Autodesk Inventor part; units mm, degrees
ref_plane "YZ Plane" through (0, 0, 0) normal (1, 0, 0) x (0, 1, 0)
ref_plane "XZ Plane" through (0, 0, 0) normal (0, 1, 0) x (-1, 0, 0)
ref_plane "XY Plane" through (0, 0, 0) normal (0, 0, 1) x (1, 0, 0)
sketch "Sketch1" plane through (0, 0, 0) normal (0, 0, 1) x (1, 0, 0)
  line L0 (0, 0) -> (7.0104, 0)
  line L1 (7.0104, 0) -> (7.0104, 3.9878)
  line L2 (7.0104, 3.9878) -> (0, 3.9878)
  line L3 (0, 3.9878) -> (0, 0)
  dimension "d0" = 7.0104
  dimension "d1" = 3.9878
extrude "Extrusion1" add sketch "Sketch1" against normal blind 1.0922
sketch "Sketch2" plane through (0, 0, -1.0922) normal (0, 0, -1) x (-1, 0, 0)
  line L0 (-7.0104, 0) -> (-7.0104, 3.9878)
  line L1 (-7.0104, 3.9878) -> (0, 3.9878)
  line L2 (-6.0071, 0.8001) -> (-1.0033, 0.8001)
  line L3 (-1.0033, 0.8001) -> (-1.0033, 3.1877)
  line L4 (-1.0033, 3.1877) -> (-6.0071, 3.1877)
  line L5 (-6.0071, 3.1877) -> (-6.0071, 0.8001)
  point P0 (-3.5052, 3.1877)
  point P1 (-3.5052, 3.9878)
  point P2 (-6.0071, 1.9939)
  point P3 (-7.0104, 1.9939)
  dimension "d4" = 5.0038
  dimension "d5" = 2.3876
extrude "Extrusion2" add sketch "Sketch2" along normal blind 1.4986
pattern_linear "Rectangular Pattern1" count 2 spacing 2.5908 along (0, 0, -1) of "Extrusion1"
sketch "Sketch3" plane through (0, 0, 0) normal (0, 0, 1) x (1, 0, 0)
  line L0 (6.0071, 3.1877) -> (1.0033, 3.1877)
  line L1 (1.0033, 3.1877) -> (1.0033, 0.8001)
  line L2 (1.0033, 0.8001) -> (6.0071, 0.8001)
  line L3 (6.0071, 0.8001) -> (6.0071, 3.1877)
  line L4 (7.0104, 3.9878) -> (0, 3.9878)
  line L5 (0, 3.9878) -> (0, 0)
  line L6 (0.6096, 0.4953) -> (6.4008, 0.4953)
  line L7 (6.4008, 0.4953) -> (6.4008, 3.4925)
  line L8 (6.4008, 3.4925) -> (0.6096, 3.4925)
  line L9 (0.6096, 3.4925) -> (0.6096, 0.4953)
  point P0 (3.5052, 3.4925)
  point P1 (3.5052, 3.9878)
  point P2 (0.6096, 1.9939)
  point P3 (0, 1.9939)
  dimension "d14" = 5.7912
  dimension "d15" = 2.9972
sketch "Sketch3 outline for Extrusion3" plane through (0, 0, 0) normal (0, 0, 1) x (1, 0, 0)
  line L0 (0.6096, 3.4925) -> (0.6096, 0.4953)
  line L1 (6.4008, 3.4925) -> (0.6096, 3.4925)
  line L2 (6.4008, 0.4953) -> (6.4008, 3.4925)
  line L3 (0.6096, 0.4953) -> (6.4008, 0.4953)
extrude "Extrusion3" add sketch "Sketch3 outline for Extrusion3" along normal blind 4.3942 draft -5
sketch "Sketch4" plane through (0, 0, 4.3942) normal (0, 0, 1) x (1, 0, 0)
  line L0 (0.994043, 0.879743) -> (0.994043, 3.108057)
  line L1 (6.016357, 0.879743) -> (0.994043, 0.879743)
  line L2 (6.016357, 3.108057) -> (6.016357, 0.879743)
  line L3 (0.994043, 3.108057) -> (6.016357, 3.108057)
  line L4 (6.025892, 3.111592) -> (0.994043, 3.111592)
  line L5 (0.994043, 3.111592) -> (0.994043, 0.879743)
  line L6 (0.994043, 0.879743) -> (6.025892, 0.879743)
  line L7 (6.025892, 0.879743) -> (6.025892, 3.111592)
  line L8 (2.860448, 1.620667) -> (2.660448, 1.620667)
  arc A0 (2.660448, 2.370667) -> (2.660448, 1.620667) centre (2.010929, 1.995667) ccw
  line L9 (2.660448, 2.370667) -> (2.860448, 2.370667)
  arc A1 (4.159487, 2.370667) -> (2.860448, 2.370667) centre (3.509967, 1.995667) ccw
  line L10 (4.159487, 2.370667) -> (4.359487, 2.370667)
  arc A2 (4.359487, 1.620667) -> (4.359487, 2.370667) centre (5.009006, 1.995667) ccw
  line L11 (4.359487, 1.620667) -> (4.159487, 1.620667)
  arc A3 (2.860448, 1.620667) -> (4.159487, 1.620667) centre (3.509967, 1.995667) ccw
  point P0 (0, 0)
extrude "Extrusion4" cut sketch "Sketch4" against normal up to next contours L8 A0 L9 A1 L10 A2 L11 A3
properties part number "276-2154" material "Rubber"
Work out the finished part from the listing and answer in its coordinate system (mm). A direction names the side the tool comes from. Give positions to 0.01 mm unless a question says otherwise; leave off trailing zeros. Write each loop counter-clockwise with the first axis right and the second up, starting at its lowest first coordinate (ties: lowest second). Pieces come first, ordered by that corner, then holes. Notation, with made-up numbers: (-11, -3.5) - (47, -3.5) arc R30 ccw to (47, 28.5) - close; hole circle Ø10 at (38, 71.25). An arc over 180 degrees is marked (long way). One line per item, written item: value. Start each with the question number.
1. Find section D-D (y = 1.5). Write down the section's boundary in (x, z), then the cut area to 3 significant figures.
2. Find section A-A (z = -3). Write down the section's boundary in (x, y).
3. Find section C-C (y = 2.9). Write down the section's boundary in (x, z).
4. For faces 5 (the flat face through (0, 2, -3)), 6 (the cylindrical face through (3.521, 2.746, 0.412)), 7 (the flat face through (6.007, 2, -2)), 8 (the flat face through (3.6, 3.988, -0.5)), 9 (the flat face through (4, 0.8, -2)), determine the directions among +Z, -Z, +X, -X, +Y, -Y from which every point of the face is accessible in a straight line to the end or side of a thin tool.
5. Consider probe 1 along X at (y, z) = (2.05, -2); probe 2 along Z at (x, y) = (5.25, 0.2); probe 3 along Y at (x, z) = (3.5, -2.25). Determine where each line is inside the solid, lowest interval first.
6. Given pin 1 (2 mm diameter, centred on x = 1.5, z = -0.5, fed in from -Y), flat-ended and moving along its own axis, determine where the tip first touches the part or whether it passes through.
7. Find section B-B (x = 3.5). Write down the section's boundary in (y, z).
8. For a pull along Z with two mould halves and no side action, classify faces 1 (the flat face through (3, 3.188, -2)), 2 (the flat face through (3.5, 0.2, 0)), 3 (the flat face through (1.003, 2, -2)), 4 (the flat face through (3.5, 0, -0.5)) as +Z half, -Z half, draft (parallel to the pull), parting line (faces both ways), or undercut.
Geometry results:
1. outline: (0, -3.68) - (1.45, -3.68) - (1.45, 4.39) - (0.99, 4.39) - (0.61, 0) - (0, 0) - (0, -1.09) - (1, -1.09) - (1, -2.59) - (0, -2.59) - close; (2.57, -3.68) - (2.95, -3.68) - (2.95, 4.39) - (2.57, 4.39) - close; (4.07, -3.68) - (4.45, -3.68) - (4.45, 4.39) - (4.07, 4.39) - close; (5.57, -3.68) - (7.01, -3.68) - (7.01, -2.59) - (6.01, -2.59) - (6.01, -1.09) - (7.01, -1.09) - (7.01, 0) - (6.4, 0) - (6.02, 4.39) - (5.57, 4.39) - close
1. area: 19.3 mm2
2. outline: (0, 0) - (7.01, 0) - (7.01, 3.99) - (0, 3.99) - close; hole (2.66, 1.62) - (2.86, 1.62) arc R0.75 ccw to (4.16, 1.62) - (4.36, 1.62) arc R0.75 ccw (long way) to (4.36, 2.37) - (4.16, 2.37) arc R0.75 ccw to (2.86, 2.37) - (2.66, 2.37) arc R0.75 ccw (long way) to start
3. outline: (0, -3.68) - (7.01, -3.68) - (7.01, -2.59) - (6.01, -2.59) - (6.01, -1.09) - (7.01, -1.09) - (7.01, 0) - (6.4, 0) - (6.02, 4.39) - (0.99, 4.39) - (0.61, 0) - (0, 0) - (0, -1.09) - (1, -1.09) - (1, -2.59) - (0, -2.59) - close
4. face 5: +Z, -Z, -X, +Y, -Y
4. face 6: +Z, -Z
4. face 7: +X, +Y, -Y
4. face 8: +Z, -Z, +X, -X, +Y
4. face 9: +X, -X, -Y
5. probe 1: 1 to 1.26, 5.76 to 6.01
5. probe 2: -3.68 to -2.59, -1.09 to 0
5. probe 3: 0.8 to 1.25, 2.75 to 3.19
6. pin 1: y = 0
7. outline: (0, -3.68) - (1.25, -3.68) - (1.25, 4.39) - (0.88, 4.39) - (0.5, 0) - (0, 0) - (0, -1.09) - (0.8, -1.09) - (0.8, -2.59) - (0, -2.59) - close; (2.75, -3.68) - (3.99, -3.68) - (3.99, -2.59) - (3.19, -2.59) - (3.19, -1.09) - (3.99, -1.09) - (3.99, 0) - (3.49, 0) - (3.11, 4.39) - (2.75, 4.39) - close
8. face 1: undercut
8. face 2: +Z half
8. face 3: undercut
8. face 4: draft
